Part print with two shaded views. Sizes in mm from the minimum x, y, z corner. Round coordinates to 2 decimals unless told otherwise and drop trailing zeros. Write each loop counter-clockwise with the first axis right and the second up, starting at its lowest first coordinate (ties: lowest second). Pieces come first, ordered by that corner, then holes. Notation, with made-up numbers: M -39,79.5 L 13,79.5 A13 ccw 13,90.5 Z; hole C 87.25,37 d10. An arc over 180 degrees is marked long. Use one line per item in the form item = value. Start each with the question number.
Item 1: Probe L1, parallel to Y at x = 3.7, z = 11. List the from-to ranges inside material, lowest first.
Item 2: Cut at A-A, the plane z = 16. Give the cut face in (x, y).
Item 3: Cut at B-B, the plane x = 3.3. Give the cut face in (y, z).
Item 4: Flat gauge pins, fed straight in: pin 1 Ø1.6 at (y, z) = (78.5, 6) entering from +X; pin 2 Ø1 at (x, z) = (2.5, 13.5) entering from -Y; pin 3 Ø1.8 at (x, z) = (3.5, 4.5) entering from +Y. Where does each tip first touch, or does it go through?
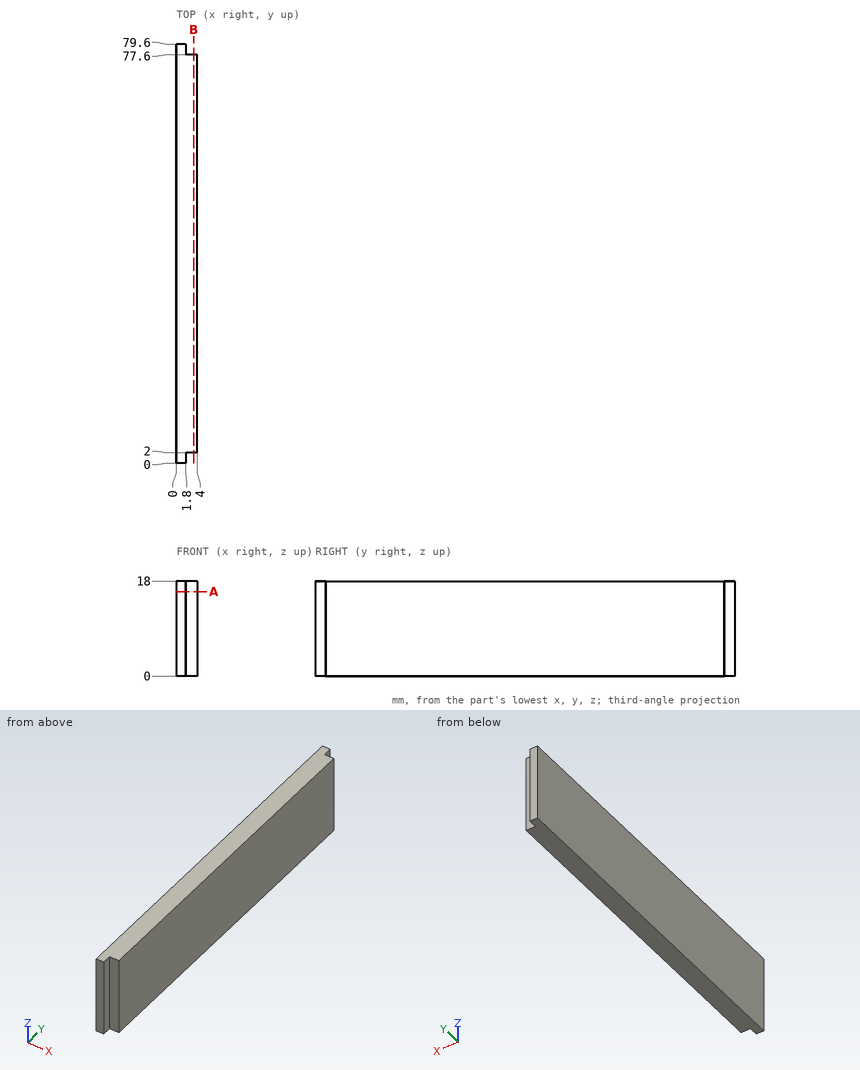
Model answer:
q1.L1 = 2 to 77.6
q2.outline = M 0,0 L 1.8,0 L 1.8,2 L 4,2 L 4,77.6 L 1.8,77.6 L 1.8,79.6 L 0,79.6 Z
q3.outline = M 2,0 L 77.6,0 L 77.6,18 L 2,18 Z
q4.pin_1 = 1.8
q4.pin_2 = 2
q4.pin_3 = 77.6
